from build123d import *

# Parameters (mm, degrees)
SKETCH_1_R          = 7.5
EXTRUDE_1_DEPTH     = 30
F_10_0MM_1_D        = 10
F_10_0MM_1_DEPTH    = 25
F_10_0MM_1_TIP      = 3.004303095
F_2_0MM_1_D         = 2
F_2_0MM_1_DEPTH     = 37
F_2_0MM_1_TIP       = 0.600860619
SKETCH_8_R          = 0.5
CUT_EXTRUDE_1_DEPTH = 44.80353867


with BuildPart() as part:
    # Sketch 1 → Extrude 1 (new body)
    with BuildSketch(Plane.XY):
        Circle(SKETCH_1_R)
    extrude(amount=EXTRUDE_1_DEPTH)

    # Sketch 2 → Revolve 1 (revolve)
    with BuildSketch(Plane(origin=(0, 0, 0), x_dir=(0, 0, -1), z_dir=(1, 0, 0)), mode=Mode.PRIVATE) as revolve_1_sk:
        with BuildLine():
            Line((-30, 0), (-30, 5.431390246))
            ThreePointArc((-30, 5.431390246), (-30.860121025, 4.119849947), (-32.405787349, 4.386048651))
            ThreePointArc((-32.405787349, 4.386048651), (-38.891100593, 5.502966287), (-42.5, 0))
            Line((-42.5, 0), (-30, 0))
        make_face()
    revolve(revolve_1_sk.sketch.rotate(Axis((0, 0, 30), (0, 0, 1)), 90), axis=Axis((0, 0, 30), (0, 0, 1)))

    # 10.0mm _1
    with Locations(Plane(origin=(0, 0, 0), x_dir=(-1, 0, 0), z_dir=(0, 0, -1))):
        with Locations((0, 0)):
            Hole(F_10_0MM_1_D / 2, depth=F_10_0MM_1_DEPTH)
            with Locations((0, 0, -(F_10_0MM_1_DEPTH + F_10_0MM_1_TIP / 2))):  # 118° drill point
                Cone(0, F_10_0MM_1_D / 2, F_10_0MM_1_TIP, mode=Mode.SUBTRACT)

    # 2.0mm _1
    with Locations(Plane(origin=(0, 0, 0), x_dir=(-1, 0, 0), z_dir=(0, 0, -1))):
        with Locations((0, 0)):
            Hole(F_2_0MM_1_D / 2, depth=F_2_0MM_1_DEPTH)
            with Locations((0, 0, -(F_2_0MM_1_DEPTH + F_2_0MM_1_TIP / 2))):  # 118° drill point
                Cone(0, F_2_0MM_1_D / 2, F_2_0MM_1_TIP, mode=Mode.SUBTRACT)

    # Sketch 8 → Cut-Extrude 1 (cut, through all)
    with BuildSketch(Plane(origin=(0, 0, 0), x_dir=(-1, 0, 0), z_dir=(0, 0, -1))):
        Circle(SKETCH_8_R)
    extrude(amount=-CUT_EXTRUDE_1_DEPTH, mode=Mode.SUBTRACT)


solid = part.part
Geometry: final body of the model. Coordinates: model frame, mm. A direction names the side the tool comes from. Round coordinates to 2 decimals unless told otherwise and drop trailing zeros. Write each loop counter-clockwise with the first axis right and the second up, starting at its lowest first coordinate (ties: lowest second). Pieces come first, ordered by that corner, then holes. Notation, with made-up numbers: M -29,88.5 L 16,88.5 A30 cw 16,121.5 Z; hole C 46,28 d9. An arc over 180 degrees is marked long. Write item = value, one per line.
Item 1: Material intervals for line 1 along Y through (x, z) = (0, 18); line 2 along Z through (x, y) = (-5.5, 5); line 3 along Z through (x, y) = (3.5, -2.25), sorted ascending. Write a range as [from, to].
Findings:
line_1 = [-7.5, -5], [5, 7.5]
line_2 = [0, 30]
line_3 = [25.5, 30.77], [32.09, 40.82]
Item 2: Section query C-C on z = 5. Return loops of the section in (x, y), then the cut area to 3 significant figures.
Findings:
outline = C 0,0 d15; hole C 0,0 d10
area = 98.2 mm^2
Item 3: Section query A-A on y = 0. Return loops of the section in (x, z), then the cut area to 3 significant figures.
Findings:
outline = M -7.5,0 L -5,0 L -5,25 L -1,27.4 L -1,37 L -0.5,37.3 L -0.5,42.48 A6 ccw -4.39,32.41 A1.43 cw -5.43,30 L -7.5,30 Z; M 0.5,37.3 L 1,37 L 1,27.4 L 5,25 L 5,0 L 7.5,0 L 7.5,30 L 5.43,30 A1.43 cw 4.39,32.41 A6 ccw 0.5,42.48 Z
area = 283 mm^2
Item 4: Pin query (flat end, axial travel): P1, Ø5, axis at x = -5, z = 5.5, coming from the -Y side; P2, Ø8, axis at y = -1, z = 16.5, coming from the -X side; P3, Ø4, axis at x = -3, y = 4, coming from the +Z side; P4, Ø4, axis at x = -5, y = -1.5, coming from the +Z side. Return the tip coordinate at first contact, or that it passes through.
Findings:
P1 = -7.07
P2 = -7.5
P3 = 41.7
P4 = 41.56
Item 5: Access query for faces 4 (the face through (-1.08, -4.88, 12.67)), 5 (the face through (2, -5, 0)). Directions: +Z, -Z, +X, -X, +Y, -Y. A direction counts if a zero-diameter tool reaches every point of the face in a straight line with its end or side. Return the directions, or none.
Findings:
face_4 = -Z
face_5 = -Z, +X, -X, +Y, -Y
Item 6: Pull-direction query (Y, two-part tool) for faces 1 (the face through (4, 4, 30)), 2 (the face through (0.108, -0.488, 39.854)), 3 (the face through (-7.493, 0.33, 14.79)); classes: pulls with the +Y half, pulls with the -Y half, needs draft (parallel to the pull), parting line crosses it, or undercut.
Findings:
face_1 = needs draft
face_2 = undercut
face_3 = parting line crosses it
